Model file for the job. Use its own axes, mm. Face numbers are marked on the shaded views. A direction names the side the tool comes from. Round coordinates to 2 decimals unless told otherwise and drop trailing zeros. Order: outer loops, then holes, each group sorted by start corner. A loop starts at its lowest first (then second) coordinate and runs counter-clockwise, first axis right, second up. Notation, with made-up numbers: (-7.75, -24.5) - (42.25, -24.5) arc R29 cw to (42.25, 11.5) - close; hole circle Ø2 at (83.25, -2). An arc over 180 degrees is marked (long way). Write item = value, one per line.
```python
from build123d import *

# Parameters (mm, degrees)
F0_W     = 66
F0_H     = 54
F1_DEPTH = 46
F2_R     = 17
F3_DEPTH = 54
F4_W     = 24
F4_H     = 16
F5_DEPTH = 66


with BuildPart() as f1:
    # F0 (on Top) → F1 (new body)
    with BuildSketch(Plane.XY):
        with Locations((11.851974, -18.000006)):
            Rectangle(F0_W, F0_H)
    extrude(amount=F1_DEPTH)

    # F2 (on face) → F3 (cut)
    with BuildSketch(Plane.XZ.offset(45.000006)):
        with Locations((11.69408, 23.092108)):
            Circle(F2_R)
    extrude(amount=-F3_DEPTH, mode=Mode.SUBTRACT)

    # F4 (on face) → F5 (cut)
    with BuildSketch(Plane.YZ.offset(44.851974)):
        with Locations((-18.06908, 22.506579)):
            Rectangle(F4_W, F4_H)
    extrude(amount=-F5_DEPTH, mode=Mode.SUBTRACT)


solid = f1.part
```
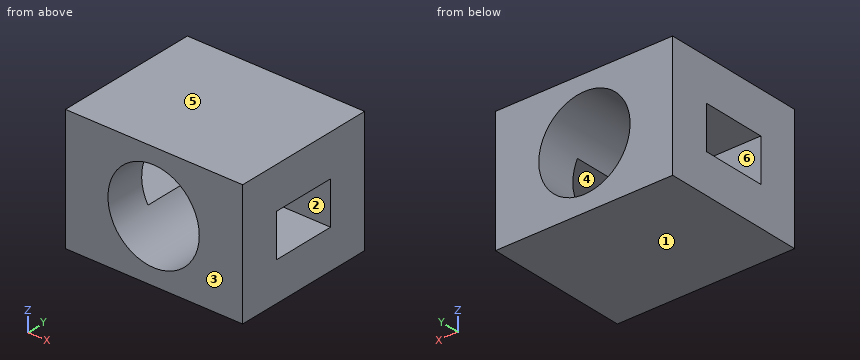
1) Cut at D-D (z = 10). Write the cut outline in (x, y), and give its area (3 significant figures).
Conclusion:
outline = (-21.15, -45) - (0.85, -45) - (0.85, 9) - (-21.15, 9) - close; (22.54, -45) - (44.85, -45) - (44.85, 9) - (22.54, 9) - close
area = 2,390 mm^2
2) 3-axis set-ups, long thin cutter, end or side, ignore diameter. For the marked faces 5 and 6: which of +Z, -Z, +X, -X, +Y, -Y reach the whole face in a straight line?
Conclusion:
face_5 = +Z, +X, -X, +Y, -Y
face_6 = +X, -X
3) Mould opens along Y. For the marked faces 1, 2, 3 and 4 say: +Y half, -Y half, draft (parallel to the pull), parting line (faces both ways), or undercut.
Conclusion:
face_1 = draft
face_2 = undercut
face_3 = -Y half
face_4 = undercut
4) Cut at C-C (x = 7). Write the cut outline in (y, z), and give its area (3 significant figures).
Conclusion:
outline = (-45, 0) - (9, 0) - (9, 6.75) - (-45, 6.75) - close; (-45, 39.43) - (9, 39.43) - (9, 46) - (-45, 46) - close
area = 719 mm^2
5) Wall check: line 1 along Y through (x, z) = (-10.5, 16.5); line 2 along Z through (x, y) = (37.5, -15); line 3 along X through (y, z) = (-19, 11). Give the ranges that are in metal, low to high.
Conclusion:
line_1 = -45 to -30.07, -6.07 to 9
line_2 = 0 to 14.51, 30.51 to 46
line_3 = -21.15 to -0.26, 23.64 to 44.85
6) Cut at B-B (z = 28). Write the cut outline in (x, y), and give its area (3 significant figures).
Conclusion:
outline = (-21.15, -45) - (-4.58, -45) - (-4.58, -30.07) - (-21.15, -30.07) - close; (-21.15, -6.07) - (-4.58, -6.07) - (-4.58, 9) - (-21.15, 9) - close; (27.97, -45) - (44.85, -45) - (44.85, -30.07) - (27.97, -30.07) - close; (27.97, -6.07) - (44.85, -6.07) - (44.85, 9) - (27.97, 9) - close
area = 1,000 mm^2
7) Cut at A-A (y = -27). Write the cut outline in (x, z), and give its area (3 significant figures).
Conclusion:
outline = (-21.15, 0) - (44.85, 0) - (44.85, 14.51) - (26.37, 14.51) arc R17 cw to (-2.98, 14.51) - (-21.15, 14.51) - close; (-21.15, 30.51) - (-3.6, 30.51) arc R17 cw to (26.99, 30.51) - (44.85, 30.51) - (44.85, 46) - (-21.15, 46) - close
area = 1,590 mm^2
